from build123d import *

# Parameters (mm, degrees)
F0_R      = 15
F1_DEPTH  = 28
F1_FACE_R = 15
F2_DEPTH  = 28
F3_R      = 15
F4_DEPTH  = 28


with BuildPart() as f1:
    # F0 (on Front) → F1 (new body)
    with BuildSketch(Plane.XZ):
        Circle(F0_R)
    extrude(amount=F1_DEPTH)

    # F1_face (on face) → F2 (join)
    with BuildSketch(Plane(origin=(0, 0, 0), x_dir=(1, 0, 0), z_dir=(0, 1, 0))):
        Circle(F1_FACE_R)
    extrude(amount=F2_DEPTH)

    # F3 (on Right) → F4 (join)
    with BuildSketch(Plane.YZ):
        Circle(F3_R)
    extrude(amount=F4_DEPTH)


solid = f1.part
CAD build for the part. Positions are in the model's coordinates, mm. A direction names the side the tool comes from. Round coordinates to 2 decimals unless told otherwise and drop trailing zeros. Write each loop counter-clockwise with the first axis right and the second up, starting at its lowest first coordinate (ties: lowest second). Pieces come first, ordered by that corner, then holes.
(1) Slice it at A-A, the plane z = 0. Write the cut outline in (x, y).
(2) Slice it at D-D, the plane z = 10.75. Write the cut outline in (x, y).
(3) Mould opens along Y. For faces 1 (the face through (0, 28, 0)), 2 (the face through (0, -28, 0)), 3 (the face through (28, 0, 0)) say: pulls with the +Y half, pulls with the -Y half, needs draft (parallel to the pull), parting line crosses it, or undercut.
(4) Slice it at C-C, the plane x = 19.5. Write the cut outline in (y, z).
(5) Drop flat-ended pins along their axis: P1, Ø5, axis at y = 17.5, z = -8, coming from the -X side; P2, Ø6, axis at y = -19.5, z = -5.5, coming from the -X side; P3, Ø5, axis at x = 16, y = -8.5, coming from the -Z side; P4, Ø6, axis at x = 2, y = -14, coming from the +Z side. Give the stop position or say it passes through.
(6) Slice it at B-B, the plane y = 0. Write the cut outline in (x, z).
(7) 3-axis set-ups, long thin cutter, end or side, ignore diameter. For faces 4 (the face through (16.915, -3.252, -14.643)), 5 (the face through (-14.985, -0.392, -0.66)): which of +Z, -Z, +X, -X, +Y, -Y reach the whole face in a straight line?
(8) Probe line 1 along Z through (x, y) = (7, -15); line 2 along Z through (x, y) = (-7.5, -23.5); line 3 along Y through (x, z) = (17.5, 8.75). List the from-to ranges inside material, lowest first.
From the geometry:
1. outline: (-15, -28) - (15, -28) - (15, -15) - (28, -15) - (28, 15) - (15, 15) - (15, 28) - (-15, 28) - close
2. outline: (-10.46, -28) - (10.46, -28) - (10.46, -10.46) - (28, -10.46) - (28, 10.46) - (10.46, 10.46) - (10.46, 28) - (-10.46, 28) - close
3. face 1: pulls with the +Y half
3. face 2: pulls with the -Y half
3. face 3: needs draft
4. outline: circle Ø30 at (0, 0)
5. P1: stops at x = -13.96
5. P2: stops at x = -14.79
5. P3: stops at z = -13.75
5. P4: stops at z = 15
6. outline: (0, -15) - (28, -15) - (28, 15) - (0, 15) arc R15 ccw to start
7. face 4: +X
7. face 5: none
8. line 1: z = -13.27 to 13.27
8. line 2: z = -12.99 to 12.99
8. line 3: y = -12.18 to 12.18
